Autodesk Inventor part; units mm, degrees
ref_plane "YZ Plane" through (0, 0, 0) normal (1, 0, 0) x (0, 1, 0)
ref_plane "XZ Plane" through (0, 0, 0) normal (0, 1, 0) x (-1, 0, 0)
ref_plane "XY Plane" through (0, 0, 0) normal (0, 0, 1) x (1, 0, 0)
sketch "Sketch1" plane through (0, 0, 0) normal (0, 1, 0) x (-1, 0, 0)
  line L0 (0, 0) -> (0, -43)
  line L1 (0, -43) -> (43, -43)
  line L2 (43, -43) -> (43, 0)
  line L3 (43, 0) -> (0, 0)
  dimension "d0" = 43
  dimension "d1" = 43
extrude "Extrusion1" add sketch "Sketch1" along normal blind 1
sketch "Sketch2" plane through (0, 1, 0) normal (0, 1, 0) x (1, 0, 0)
  line L0 (-43, 0) -> (0, 0)
  line L1 (0, 0) -> (-3, 0)
  line L2 (-3, 0) -> (-3, 3)
  line L3 (-3, 3) -> (0, 3)
  circle A0 centre (-3, 3) radius 1.5
  line L4 (0, 43) -> (-43, 43)
  line L5 (0, 0) -> (-43, 43)
  line L6 (-43, 43) -> (-43, 0)
  line L7 (-43, 43) -> (-43, 0)
  line L8 (0, 0) -> (0, 43)
  line L9 (-43, 0) -> (0, 43)
  line L10 (0, 43) -> (-21.5, 21.5)
  circle A1 centre (-3, 40) radius 1.5
  circle A2 centre (-40, 40) radius 1.5
  circle A3 centre (-40, 3) radius 1.5
  dimension "d4" = 3
  dimension "d5" = 3
  dimension "d6" = 3
  dimension "d9" = 360
extrude "Extrusion2" cut sketch "Sketch2" against normal through all contours A3 L9 | L9 A3 | A0 L5 L2 | L2 L5 A0 | A2 L5 | L5 A2 | L5 L3 A0 | L5 A0 L3 | A1 L9 | L9 A1
sketch "Sketch3" plane through (0, 1, 0) normal (0, 1, 0) x (1, 0, 0)
  line L0 (-43, 0) -> (0, 0)
  line L1 (0, 0) -> (0, 10)
  line L2 (0, 0) -> (0, 43)
  line L3 (0, 10) -> (0, 43)
  line L4 (0, 43) -> (0, 33)
  line L5 (0, 33) -> (0, 10)
  line L6 (0, 10) -> (-15, 10)
  line L7 (-15, 10) -> (-15, 33)
  line L8 (-15, 33) -> (0, 33)
  line L9 (0, 10) -> (0, 14.4)
  line L10 (0, 14.4) -> (0, 18.8)
  line L11 (0, 33) -> (0, 28.6)
  line L12 (0, 28.6) -> (0, 24.2)
  line L13 (0, 24.2) -> (0, 18.8)
  line L14 (0, 14.4) -> (0, 15)
  line L15 (0, 33) -> (0, 32.6)
  line L16 (0, 32.6) -> (-15, 32.6)
  line L17 (0, 32.6) -> (0, 28.6)
  line L18 (0, 28.6) -> (-15, 28.6)
  line L19 (0, 28.6) -> (0, 28.2)
  line L20 (0, 28.2) -> (-15, 28.2)
  line L21 (0, 28.2) -> (0, 24.2)
  line L22 (0, 18.8) -> (0, 24.2)
  line L23 (0, 32.6) -> (0, 28.6)
  line L24 (0, 28.2) -> (0, 24.2)
  line L25 (0, 24.2) -> (-15, 24.2)
  line L26 (0, 24.2) -> (0, 23.8)
  line L27 (0, 23.8) -> (-15, 23.8)
  line L28 (0, 18.8) -> (0, 19.2)
  line L29 (0, 19.2) -> (-15, 19.2)
  line L30 (0, 18.8) -> (-15, 18.8)
  line L31 (0, 14.4) -> (-15, 14.4)
  line L32 (0, 10) -> (0, 10.4)
  line L33 (0, 10.4) -> (-15, 10.4)
  line L34 (0, 10.4) -> (0, 14.4)
  line L35 (0, 14.4) -> (0, 14.8)
  line L36 (0, 14.8) -> (-15, 14.8)
  line L37 (0, 10) -> (-7.5, 10)
  line L38 (-7.5, 10) -> (-7.5, 33)
  line L39 (-7.5, 10) -> (-7.7, 10)
  line L40 (-7.7, 10) -> (-7.3, 10)
  line L41 (-7.3, 10) -> (-7.3, 33)
  line L42 (-7.7, 10) -> (-7.7, 33)
  point P0 (-7.7, 10.4)
  point P1 (-7.3, 10.4)
  point P2 (-7.3, 14.4)
  point P3 (-7.3, 14.8)
  point P4 (-7.3, 18.8)
  point P5 (-7.3, 19.2)
  point P6 (-7.3, 23.8)
  point P7 (-7.3, 24.2)
  point P8 (-7.3, 28.2)
  point P9 (-7.3, 28.6)
  point P10 (-7.3, 32.6)
  point P11 (-7.7, 32.6)
  dimension "d13" = 10
  dimension "d14" = 10
  dimension "d15" = 23
  dimension "d16" = 15
  dimension "d17" = 4.4
  dimension "d18" = 4.4
  dimension "d19" = 4.4
  dimension "d20" = 4.4
  dimension "d22" = 0.4
  dimension "d23" = 0.4
  dimension "d24" = 0.4
  dimension "d25" = 0.4
  dimension "d26" = 0.4
  dimension "d27" = 0.4
  dimension "d28" = 0.2
  dimension "d29" = 0.4
extrude "Extrusion3" add sketch "Sketch3" along normal blind 24 contours L6 L41 L33 L2 | L6 L38 L33 L41 | L31 L41 L36 L2 | L33 L38 L31 L41 | L6 L42 L33 L38 | L31 L38 L36 L41 | L33 L42 L31 L38 | L6 L7 L33 L42 | L36 L38 L30 L41 | L31 L42 L36 L38 | L30 L41 L29 L2 | L36 L42 L30 L38 | L30 L38 L29 L41 | L30 L42 L29 L38 | L29 L38 L27 L41 | L27 L41 L25 L2 | L29 L42 L27 L38 | L27 L38 L25 L41 | L27 L42 L25 L38 | L25 L38 L20 L41 | L20 L41 L18 L2 | L25 L42 L20 L38 | L20 L38 L18 L41 | L20 L42 L18 L38 | L18 L38 L16 L41 | L16 L41 L8 L2 | L18 L42 L16 L38 | L16 L38 L8 L41 | L16 L42 L8 L38 | L16 L7 L8 L42
properties part number "L298N"
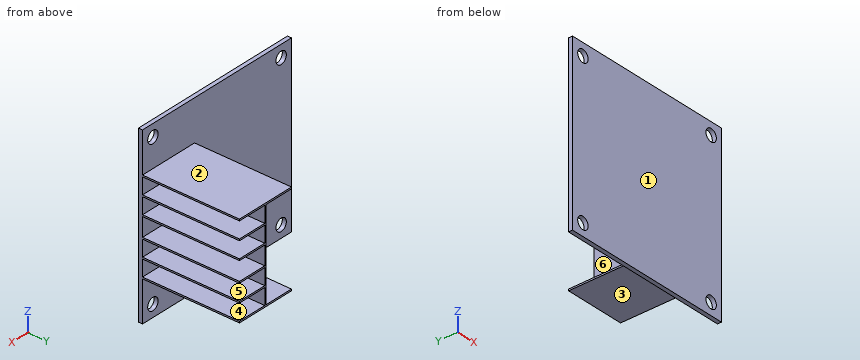
Check sheet for the modelled part. Datum: model origin and axes. Units: mm. Face numbers are marked on the shaded views. A direction names the side the tool comes from. Give positions to 0.01 mm unless a question says otherwise; leave off trailing zeros. Loops run counter-clockwise (first coordinate to the right, second up) from the corner with the lowest first, then second, coordinate; pieces in that order, holes last. Notation, with made-up numbers: M 30.5,74.5 L 86.5,74.5 A24 ccw 86.5,89.5 Z; hole C 73,35.5 d6. An arc over 180 degrees is marked long. Answer in a Markdown table with one row per item.
1) Cross-section at C-C (y = 16.25). Enter the section's corners in (x, z), plus the area to 3 significant figures.
Solutions:
| item | result |
|---|---|
| outline | M -15,-33 L 0,-33 L 0,-32.6 L -7.3,-32.6 L -7.3,-28.6 L 0,-28.6 L 0,-28.2 L -7.3,-28.2 L -7.3,-24.2 L 0,-24.2 L 0,-23.8 L -7.3,-23.8 L -7.3,-19.2 L 0,-19.2 L 0,-18.8 L -7.3,-18.8 L -7.3,-14.8 L 0,-14.8 L 0,-14.4 L -7.3,-14.4 L -7.3,-10.4 L 0,-10.4 L 0,-10 L -15,-10 L -15,-10.4 L -7.7,-10.4 L -7.7,-32.6 L -15,-32.6 Z |
| area | 32.6 mm^2 |
2) Cross-section at D-D (z = -32). Enter the section's corners in (x, y).
Solutions:
| item | result |
|---|---|
| outline | M -43,0 L 0,0 L 0,1 L -7.3,1 L -7.3,25 L -7.7,25 L -7.7,1 L -43,1 Z |
3) Cross-section at B-B (x = -40). Enter the section's corners in (y, z), plus the area to 3 significant figures.
Solutions:
| item | result |
|---|---|
| outline | M 0,-43 L 1,-43 L 1,-41.5 L 0,-41.5 Z; M 0,-38.5 L 1,-38.5 L 1,-4.5 L 0,-4.5 Z; M 0,-1.5 L 1,-1.5 L 1,0 L 0,0 Z |
| area | 37.0 mm^2 |
4) Depth check by flat-ended pin: pin 1 (8 mm diameter, centred on x = -2.5, y = 18, fed in from +Z); pin 2 (3.5 mm diameter, centred on x = -11, y = 16, fed in from -Z); pin 3 (6 mm diameter, centred on y = 12.5, z = -32.5, fed in from -X). Enter the tip coordinate at first touch or a pass-through.
Solutions:
| item | result |
|---|---|
| pin 1 | stops at z = -10 |
| pin 2 | stops at z = -33 |
| pin 3 | stops at x = -15 |
5) Mould release check, pull along Z, two halves, no side actions. Record for the marked faces 1, 2, 3 and 4: released by +Z, released by -Z, zero draft, split by the parting line, or undercut.
Solutions:
| item | result |
|---|---|
| face 1 | zero draft |
| face 2 | released by +Z |
| face 3 | released by -Z |
| face 4 | undercut |
6) Tool access check on the marked faces 5 and 6. Record the directions out of +Z, -Z, +X, -X, +Y, -Y that give a thin tool (end or side, any length) a straight path to the whole face; none if there is none.
Solutions:
| item | result |
|---|---|
| face 5 | +X, +Y |
| face 6 | -X, +Y |
7) Thickness scan on line 1 (X direction, y = 0.25, z = -40); line 2 (Z direction, x = -4, y = 2.75). Record the ranges inside material, lowest first.
Solutions:
| item | result |
|---|---|
| line 1 | x = -43 to -41.5, -38.5 to -4.5, -1.5 to 0 |
| line 2 | z = -33 to -32.6, -28.6 to -28.2, -24.2 to -23.8, -19.2 to -18.8, -14.8 to -14.4, -10.4 to -10 |
8) Cross-section at A-A (z = -3). Enter the section's corners in (x, y).
Solutions:
| item | result |
|---|---|
| outline | M -43,0 L -41.5,0 L -41.5,1 L -43,1 Z; M -38.5,0 L -4.5,0 L -4.5,1 L -38.5,1 Z; M -1.5,0 L 0,0 L 0,1 L -1.5,1 Z |
